Autodesk Inventor part; units mm, degrees
ref_plane "YZ Plane" through (0, 0, 0) normal (1, 0, 0) x (0, 1, 0)
ref_plane "XZ Plane" through (0, 0, 0) normal (0, 1, 0) x (-1, 0, 0)
ref_plane "XY Plane" through (0, 0, 0) normal (0, 0, 1) x (1, 0, 0)
sketch "Sketch1" plane through (0, 0, 0) normal (0, 0, 1) x (1, 0, 0)
  line L0 (12.7, 0) -> (266.7, 0)
  line L1 (279.4, 12.7) -> (279.4, 88.9)
  line L2 (266.7, 101.6) -> (12.7, 101.6)
  line L3 (0, 88.9) -> (0, 12.7)
  arc A0 (12.7, 101.6) -> (0, 88.9) centre (12.7, 88.9) ccw
  arc A1 (0, 12.7) -> (12.7, 0) centre (12.7, 12.7) ccw
  arc A2 (266.7, 0) -> (279.4, 12.7) centre (266.7, 12.7) ccw
  arc A3 (279.4, 88.9) -> (266.7, 101.6) centre (266.7, 88.9) ccw
  point P0 (0, 0)
  point P1 (279.4, 101.6)
  point P2 (279.4, 0)
  point P3 (0, 101.6)
  dimension "d0" = 279.4
  dimension "d1" = 101.6
  dimension "d2" = 12.7
extrude "Extrusion1" add sketch "Sketch1" along normal blind 12.7
chamfer "Chamfer1" distance 0.7937 angle 45 16 edges at (139.7, 101.6, 12.7) (3.7197, 97.8803, 12.7) (0, 50.8, 12.7) (3.7197, 3.7197, 12.7) (139.7, 0, 12.7) (275.6803, 3.7197, 12.7) (279.4, 50.8, 12.7) (275.6803, 97.8803, 12.7) (139.7, 101.6, 0) (3.7197, 97.8803, 0) (0, 50.8, 0) (3.7197, 3.7197, 0) (139.7, 0, 0) (275.6803, 3.7197, 0) (279.4, 50.8, 0) (275.6803, 97.8803, 0)
sketch "Sketch2" plane through (0, 0, 12.7) normal (0, 0, 1) x (1, 0, 0)
  line L0 (0.7937, 12.7) -> (0.7938, 88.9)
  line L1 (0, 88.9) -> (0, 12.7)
  line L2 (266.7, 101.6) -> (12.7, 101.6)
  line L3 (279.4, 12.7) -> (279.4, 88.9)
  point P0 (0, 0)
  point P1 (11.1125, 50.8)
  point P2 (38.1, 50.8)
  point P3 (139.7, 50.8)
  point P4 (268.2875, 50.8)
  dimension "d9" = 11.1125
  dimension "d10" = 50.8
  dimension "d11" = 50.8
  dimension "d12" = 50.8
  dimension "d13" = 50.8
  dimension "d14" = 11.1125
  dimension "d15" = 139.7
  dimension "d16" = 38.1
hole "Hole1" at (11.1125, 50.8, 12.7) at (268.2875, 50.8, 12.7) direction (0, 0, -1) diameter 6.35 end through all countersink diameter 12.7 countersink angle 82
hole "Hole2" at (38.1, 50.8, 12.7) at (139.7, 50.8, 12.7) direction (0, 0, -1) diameter 7.9375 end through all
sketch "Sketch3" plane through (0, 0, 0) normal (0, 0, -1) x (-1, 0, 0)
  arc A0 (-12.7, 0.7937) -> (-0.7938, 12.7) centre (-12.7, 12.7) ccw
  arc A1 (-0.7938, 88.9) -> (-12.7, 100.8062) centre (-12.7, 88.9) ccw
  arc A2 (-266.7, 100.8062) -> (-278.6063, 88.9) centre (-266.7, 88.9) ccw
  arc A3 (-278.6063, 12.7) -> (-266.7, 0.7938) centre (-266.7, 12.7) ccw
  point P0 (0, 0)
hole "Hole3" at (12.7, 12.7, 0) at (12.7, 88.9, 0) at (266.7, 88.9, 0) at (266.7, 12.7, 0) direction (0, 0, 1) diameter 3.302 depth 7.3025
properties part number "Base Plate"
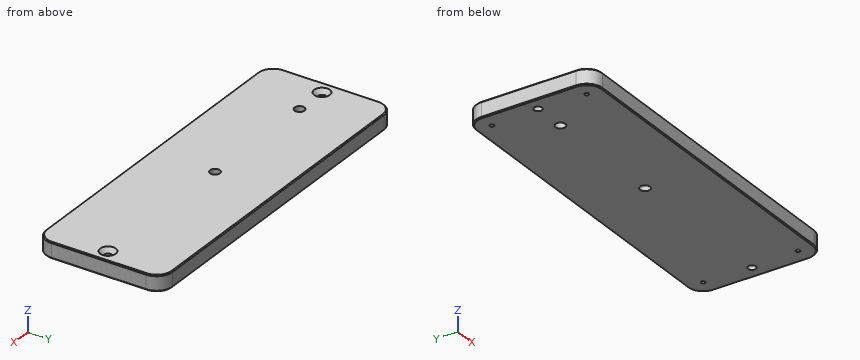
Part model, mm, in its own coordinate system. Coordinates: 2 decimals unless noted, no trailing zeros. Order: outer loops, then holes, each group sorted by start corner. A loop starts at its lowest first (then second) coordinate and runs counter-clockwise, first axis right, second up. Notation, with made-up numbers: (60, 80) -> (117, 80) arc R25 cw to (117, 97) -> close; hole circle Ø7 at (37.25, 14). An arc over 180 degrees is marked (long way). Put each result on its own line as item: value. Start each with the question number.
(1) Pin check, flat tip, straight feed: pin 1 Ø2.5 at (x, y) = (12.7, 88.9) entering from -Z. Stop position of the tip, or through.
(2) Band-saw the part on A-A (x = 139.7). Give the cut face in (y, z).
(3) Probe line 1 along X through (y, z) = (50.8, 4.5); line 2 along X through (y, z) = (88.9, 6.25); line 3 along Y through (x, z) = (266.7, 2.5). List the from-to ranges inside material, lowest first. Write a range as [from, to].
(4) Band-saw the part on B-B (y = 50.8). Give the cut face in (x, z).
Determined:
1. pin 1: stops at z = 7.3
2. outline: (0, 0.79) -> (0.79, 0) -> (46.83, 0) -> (46.83, 12.7) -> (0.79, 12.7) -> (0, 11.91) -> close; (54.77, 0) -> (100.81, 0) -> (101.6, 0.79) -> (101.6, 11.91) -> (100.81, 12.7) -> (54.77, 12.7) -> close
3. line 1: x = [0, 7.94], [14.29, 34.13], [42.07, 135.73], [143.67, 265.11], [271.46, 279.4]
3. line 2: x = [0, 11.05], [14.35, 265.05], [268.35, 279.4]
3. line 3: y = [0, 11.05], [14.35, 48.05], [53.55, 87.25], [90.55, 101.6]
4. outline: (0, 0.79) -> (0.79, 0) -> (7.94, 0) -> (7.94, 9.05) -> (4.76, 12.7) -> (0.79, 12.7) -> (0, 11.91) -> close; (14.29, 0) -> (34.13, 0) -> (34.13, 12.7) -> (17.46, 12.7) -> (14.29, 9.05) -> close; (42.07, 0) -> (135.73, 0) -> (135.73, 12.7) -> (42.07, 12.7) -> close; (143.67, 0) -> (265.11, 0) -> (265.11, 9.05) -> (261.94, 12.7) -> (143.67, 12.7) -> close; (271.46, 0) -> (278.61, 0) -> (279.4, 0.79) -> (279.4, 11.91) -> (278.61, 12.7) -> (274.64, 12.7) -> (271.46, 9.05) -> close
